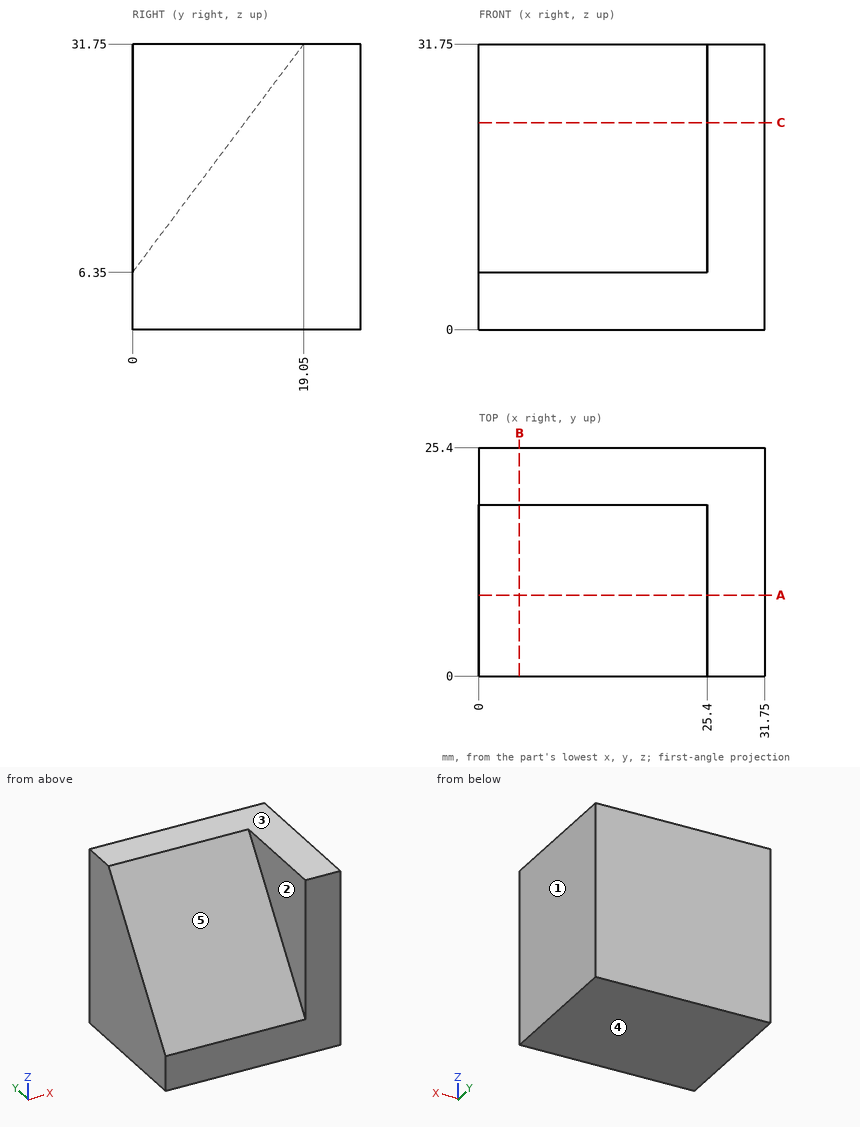
The figure shows three views and two pictorial views of one solid part (mm, origin at its lowest corner). Answer the questions. A direction names the side the tool comes from. Give positions to 0.01 mm unless a question says otherwise; leave off trailing zeros. Write each loop counter-clockwise with the first axis right and the second up, starting at its lowest first coordinate (ties: lowest second). Pieces come first, ordered by that corner, then holes.
Q1. Straight lines are drawn through the part: L1, parallel to X at y = 6.25, z = 23.5; L2, parallel to Z at x = 22, y = 15.5; L3, parallel to Y at x = 12, z = 12. For each, find the intervals that lie inside material, in ascending order.
Answer:
L1: x = 25.4 to 31.75
L2: z = 0 to 27.02
L3: y = 4.24 to 25.4
Q2. The part is cut by section C-C on z = 23. Give the vertices of the cut face in (x, y).
Answer:
outline: (0, 12.49) - (25.4, 12.49) - (25.4, 0) - (31.75, 0) - (31.75, 25.4) - (0, 25.4) - close
Q3. A tool of negligible diameter and unlimited length cuts with its end or side. For the marked faces 4 and 5, from which of +Z, -Z, +X, -X, +Y, -Y can it reach the whole face along a straight path? Write none if from no direction.
Answer:
face 4: -Z, +X, -X, +Y, -Y
face 5: +Z, -X, -Y
Q4. Given pin 1 (3 mm diameter, centred on y = 22, z = 12.5, fed in from -X); pin 2 (1 mm diameter, centred on x = 24.5, z = 28, fed in from -Y), each flat-ended and moving along its own axis, determine where each tip first touches the part or whether it passes through.
Answer:
pin 1: stops at x = 0
pin 2: stops at y = 15.86
Q5. The part is cut by section B-B on x = 4.5. Give the vertices of the cut face in (y, z).
Answer:
outline: (0, 0) - (25.4, 0) - (25.4, 31.75) - (19.05, 31.75) - (0, 6.35) - close
Q6. The part is cut by section A-A on y = 9. Give the vertices of the cut face in (x, z), and give its area (3 significant figures).
Answer:
outline: (0, 0) - (31.75, 0) - (31.75, 31.75) - (25.4, 31.75) - (25.4, 18.35) - (0, 18.35) - close
area: 668 mm2
Q7. For a pull along X with two mould halves and no side action, classify the marked faces 1, 2 and 3 as released by +X, released by -X, zero draft, split by the parting line, or undercut.
Answer:
face 1: released by +X
face 2: released by -X
face 3: zero draft
